from build123d import *

# Parameters (mm, degrees)
ESQUISSE1_R        = 5
BOSS_EXTRU_1_DEPTH = 75
BOSS_EXTRU_2_DEPTH = 8


with BuildPart() as part:
    # Esquisse1 → Boss.-Extru.1 (new body)
    with BuildSketch(Plane(origin=(0, 0, 0), x_dir=(1, 0, 0), z_dir=(0, 1, 0))):
        with Locations(Location((0, 0, 0), (0, 0, 270))):
            Circle(ESQUISSE1_R)
    extrude(amount=BOSS_EXTRU_1_DEPTH)

    # Esquisse2 → Boss.-Extru.2 (add)
    with BuildSketch(Plane(origin=(0, 75, 0), x_dir=(1, 0, 0), z_dir=(0, 1, 0))):
        Polygon((-5, 8.660254038), (5, 8.660254038), (10, 0), (5, -8.660254038), (-5, -8.660254038), (-10, 0), align=None)
    extrude(amount=BOSS_EXTRU_2_DEPTH)


solid = part.part
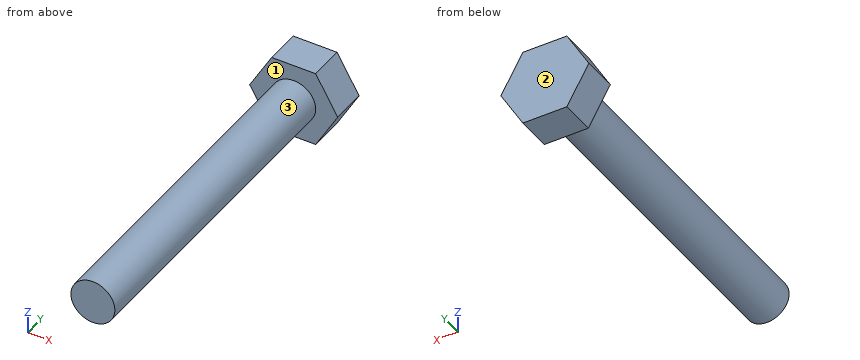
Model file for the job. Use its own axes, mm. Face numbers are marked on the shaded views. Give positions to 0.01 mm unless a question says otherwise; leave off trailing zeros. Order: outer loops, then holes, each group sorted by start corner. A loop starts at its lowest first (then second) coordinate and runs counter-clockwise, first axis right, second up. Notation, with made-up numbers: (12, -16.75) - (68, -16.75) arc R19 cw to (68, 6.25) - close; hole circle Ø10 at (-39.75, 32.25). An arc over 180 degrees is marked (long way). Write item = value, one per line. Start each with the question number.
1. Cut at B-B, the plane z = -0.75. List the corners of the cut face in (x, y), and give its area (3 significant figures).
2. Probe line 1 along Y through (x, z) = (-4, 8.25); line 2 along X through (y, z) = (50, 3); line 3 along X through (y, z) = (49, 3.75). List the from-to ranges inside material, lowest first.
3. Cut at C-C, the plane y = 54.5. List the corners of the cut face in (x, z), and give its area (3 significant figures).
4. Drop flat-ended pins along their axis: P1, Ø1.5, axis at x = 6, y = 61, coming from the -Z side; P2, Ø8, axis at x = -4.5, y = 40.5, coming from the +Z side; P3, Ø1, axis at x = -1, y = 26, coming from the -Z side; P4, Ø6, axis at y = 39.5, z = -5, coming from the -X side. Give the stop position or say it passes through.
5. Two-plate mould, pull along Y, no slides. Class the marked faces 1, 2 and 3: pulls with the +Y half, pulls with the -Y half, needs draft (parallel to the pull), parting line crosses it, or undercut.
6. Cut at A-A, the plane x = 0. List the corners of the cut face in (y, z), and give its area (3 significant figures).
7. Cut at D-D, the plane x = -8.5. List the corners of the cut face in (y, z), and give its area (3 significant figures).
Taken from the geometry:
q1.outline = (-9.57, 75) - (-4.94, 75) - (-4.94, 0) - (4.94, 0) - (4.94, 75) - (9.57, 75) - (9.57, 83) - (-9.57, 83) - close
q1.area = 895 mm²
q2.line_1 = 75 to 83
q2.line_2 = -4 to 4
q2.line_3 = -3.31 to 3.31
q3.outline = circle Ø10 at (0, 0)
q3.area = 78.5 mm²
q4.P1 = through
q4.P2 = 4.97
q4.P3 = -4.97
q4.P4 = -4.58
q5.face_1 = pulls with the -Y half
q5.face_2 = pulls with the +Y half
q5.face_3 = needs draft
q6.outline = (0, -5) - (75, -5) - (75, -8.66) - (83, -8.66) - (83, 8.66) - (75, 8.66) - (75, 5) - (0, 5) - close
q6.area = 889 mm²
q7.outline = (75, -2.6) - (83, -2.6) - (83, 2.6) - (75, 2.6) - close
q7.area = 41.6 mm²
